from build123d import *

# Parameters (mm, degrees)
F1_DEPTH = 63.5
F2_DEPTH = 25.4
F3_DEPTH = 7.9375
F4_DEPTH = 25.4
F6_R     = 6.35


# Not quite as in the source:
# - a feature names something its author has since deleted; it is built from what else it names


with BuildPart() as f1:
    # F0 (on Front) → F1 (new body, symmetric)
    with BuildSketch(Plane.XZ):
        Polygon((22.225, 9.525), (-41.275, 9.525), (-41.275, -9.525), (41.275, -9.525), (41.275, 9.525), align=None)
    extrude(amount=F1_DEPTH, both=True)

    # F0 (on Front) → F2 (join, symmetric)
    with BuildSketch(Plane.XZ):
        with BuildLine():
            Line((22.225, 27.051), (22.225, 9.525))
            Line((22.225, 9.525), (41.275, 9.525))
            Line((41.275, 9.525), (41.275, 27.051))
            ThreePointArc((41.275, 27.051), (45.9246798487, 38.2763201513), (57.15, 42.926))
            Line((57.15, 42.926), (60.325, 42.926))
            Line((60.325, 42.926), (60.325, 61.976))
            Line((60.325, 61.976), (57.15, 61.976))
            add(Edge.make_bspline(
                [(55.6844107211, 61.9452355277), (56.1739766533, 61.9576548863), (56.6625337097, 61.9679123237), (57.15, 61.976)],
                knots=[110.3317061333, 110.3317061333, 110.3317061333, 110.3317061333, 111.5284180198, 111.5284180198, 111.5284180198, 111.5284180198], degree=3))
            ThreePointArc((55.6844107211, 61.9452355277), (31.9414565021, 51.2229870866), (22.225, 27.051))
        make_face()
    extrude(amount=F2_DEPTH, both=True)

    # F0 (on Front) → F3 (join, symmetric)
    with BuildSketch(Plane.XZ):
        with BuildLine():
            add(Edge.make_bspline(
                [(-41.275, 9.525), (-43.1628450735, 41.2787763348), (10.5485303307, 60.8002239091), (55.6844107211, 61.9452355277)],
                knots=[0, 0, 0, 0, 110.3317061333, 110.3317061333, 110.3317061333, 110.3317061333], degree=3))
            Line((-41.275, 9.525), (22.225, 9.525))
            Line((22.225, 9.525), (22.225, 27.051))
            ThreePointArc((22.225, 27.051), (31.9414565021, 51.2229870866), (55.6844107211, 61.9452355277))
        make_face()
    extrude(amount=F3_DEPTH, both=True)

    # F0 (on Front) → F4 (join, symmetric)
    with BuildSketch(Plane.XZ):
        Polygon((79.1998635302, 61.976), (60.325, 61.976), (60.325, 42.926), (78.823101495, 42.926), align=None)
    extrude(amount=F4_DEPTH, both=True)

    # F0 (on Front) → F5 (revolve)
    with BuildSketch(Plane.XZ):
        Polygon((79.2927981655, 66.675), (79.1998635302, 61.976), (78.823101495, 42.926), (78.7276551127, 38.1), (111.125, 38.1), (111.125, 66.675), align=None)
    revolve(axis=Axis((79.0102266391, 0, 52.3875), (0.0197736678, 0, 0.9998044819)))

    # F6
    f6_edges = [f1.edges().sort_by_distance(p)[0] for p in [
        (41.275, -63.5, 0),
        (-41.275, -63.5, 0),
        (-41.275, 63.5, 0),
        (41.275, 63.5, 0),
    ]]
    fillet(f6_edges, radius=F6_R)


solid = f1.part
Geometry check sheet. Reference: the model listing, model coordinates, mm. A direction names the side the tool comes from. Give positions to 0.01 mm unless a question says otherwise; leave off trailing zeros. Order: outer loops, then holes, each group sorted by start corner. A loop starts at its lowest first (then second) coordinate and runs counter-clockwise, first axis right, second up.
1) Material ranges on probe 1 along X at (y, z) = (-32, 1) (3 decimals); probe 2 along Z at (x, y) = (-32, -31) (3 decimals); probe 3 along Y at (x, z) = (4, 49), recorded low to high.
Results are:
probe 1: x = -41.275 to 41.275
probe 2: z = -9.525 to 9.525
probe 3: y = -7.94 to 7.94
2) Gauge pin test, flat ends, axial feed: pin 1 (5 mm diameter, centred on y = -18.5, z = 20, fed in from -X) (3 decimals); pin 2 (1.1 mm diameter, centred on x = 58.5, y = 24.5, fed in from +Z); pin 3 (11.5 mm diameter, centred on x = 32.5, z = 35.5, fed in from -Y). Record the tip position at first contact, or that the pin passes through.
Results are:
pin 1: stops at x = 22.225
pin 2: stops at z = 67.72
pin 3: stops at y = -25.4
3) Cross-section at B-B (y = -35). Record the boundary of the cut face in (x, z) (3 decimals), then the cut area to 3 significant figures.
Results are:
outline: (-41.275, -9.525) - (41.275, -9.525) - (41.275, 9.525) - (-41.275, 9.525) - close
area: 1,570 mm2
4) Tool access check on faces 1 (the flat face through (41.275, -1, 4)), 2 (the cylindrical face through (32.2, 16.55, 51.49)), 3 (the flat face through (37, -25.4, 36)), 4 (the flat face through (0, 63.5, 0)). Record the directions out of +Z, -Z, +X, -X, +Y, -Y that give a thin tool (end or side, any length) a straight path to the whole face; none if there is none.
Results are:
face 1: -Z, +X, +Y, -Y
face 2: +Z, -X, +Y
face 3: +Z, -X, -Y
face 4: +Z, -Z, +X, -X, +Y
5) Cross-section at A-A (z = 2). Record the boundary of the cut face in (x, y) (3 decimals), then the cut area to 3 significant figures.
Results are:
outline: (-41.275, -57.15) arc R6.35 ccw to (-34.925, -63.5) - (34.925, -63.5) arc R6.35 ccw to (41.275, -57.15) - (41.275, 57.15) arc R6.35 ccw to (34.925, 63.5) - (-34.925, 63.5) arc R6.35 ccw to (-41.275, 57.15) - close
area: 10,400 mm2
6) Draft check along X on faces 5 (the flat face through (22.225, -17, 18)), 6 (the conical face through (80.7, 0.6, 38.1)), 7 (the flat face through (-7, -7.938, 30)). Enter one of: released by +X, released by -X, zero draft, split by the parting line, or undercut.
Results are:
face 5: released by -X
face 6: undercut
face 7: zero draft
